CAD build for the part. Positions are in the model's coordinates, mm. A direction names the side the tool comes from. Coordinates: 2 decimals unless noted, no trailing zeros. Loops run counter-clockwise (first coordinate to the right, second up) from the corner with the lowest first, then second, coordinate; pieces in that order, holes last. Notation, with made-up numbers: (76, -33) -> (124, -33) arc R22 cw to (124, -5) -> close; hole circle Ø7 at (24.5, 20.25). An arc over 180 degrees is marked (long way). Return JSON: item names as keys, results as strings. Group by question number.
(1) Flat gauge pins, fed straight in: pin 1 Ø4 at (x, y) = (-8.5, -72.5) entering from +Z; pin 2 Ø12 at (x, y) = (-67.5, 66) entering from +Z; pin 3 Ø1 at (y, z) = (4.5, 59.5) entering from -X; pin 4 Ø4 at (x, y) = (-84.36, -38.25) entering from -Z. Where does each tip first touch, or does it go through?
(2) Saw through at B-B on x = 77. Write the cut outline in (y, z).
(3) Saw through at D-D on z = 54.25. Give the number of separate pieces and of enclosed holes in the cut face, then the cut area to 3 significant figures.
(4) Tool access for faces 1 (the face through (-72.5, 0, 57)), 2 (the face through (-77, 48, 57)): list every direction of +Z, -Z, +X, -X, +Y, -Y with a clear straight run to the whole face (end or side of a thin tool).
(5) Saw through at A-A on y = -13.5. Write the cut outline in (x, z), then the cut area to 3 significant figures.
(6) Mould opens along Y. For faces 3 (the face through (39.16, -61.41, 56.94)), 4 (the face through (-1.588, -84.596, 54.972)) say: pulls with the +Y half, pulls with the -Y half, needs draft (parallel to the pull), parting line crosses it, or undercut.
(7) Saw through at C-C on x = 22. Write the cut outline in (y, z).
(8) Probe L1, parallel to Y at x = 77.5, z = 60.5; L2, parallel to Y at x = -67.5, z = 55; L3, parallel to Y at x = -35, z = 56. List the from-to ranges inside material, lowest first.
```python
from build123d import *

# Parameters (mm, degrees)
F0_W      = 190
F0_H      = 175
F1_DEPTH  = 8
F2_R      = 4.5
F2_R_2    = 1.6
F3_DEPTH  = 8
F5_DEPTH  = 8.001
F6_R      = 12.2
F6_R_2    = 4.5
F7_DEPTH  = 4
F8_R      = 1.7
F8_W      = 145
F8_H      = 33.2
F8_R_2    = 1.8
F9_DEPTH  = 8.001
F10_ANGLE = 180


with BuildPart() as f1:
    # F0 (on Top) → F1 (new body)
    with BuildSketch(Plane.XY):
        Rectangle(F0_W, F0_H)
    extrude(amount=F1_DEPTH)

    # F2 (on face) → F3 (cut)
    with BuildSketch(Plane.XY.offset(8)):
        with Locations((0, 72.5)):
            Circle(F2_R)
        with Locations((-77, 42.5)):
            Circle(F2_R)
        with Locations((8.5, 72.5)):
            Circle(F2_R_2)
        with Locations((-8.5, 72.5)):
            Circle(F2_R_2)
        with Locations((-84.361216, 38.25)):
            Circle(F2_R_2)
        with Locations((-69.638784, 46.75)):
            Circle(F2_R_2)
        with Locations((77, 42.5)):
            Circle(F2_R)
        with Locations((84.361216, 38.25)):
            Circle(F2_R_2)
        with Locations((69.638784, 46.75)):
            Circle(F2_R_2)
        with Locations((-84.361216, -38.25)):
            Circle(F2_R_2)
        with Locations((-77, -42.5)):
            Circle(F2_R)
        with Locations((-69.638784, -46.75)):
            Circle(F2_R_2)
        with Locations((-8.5, -72.5)):
            Circle(F2_R_2)
        with Locations((0, -72.5)):
            Circle(F2_R)
        with Locations((8.5, -72.5)):
            Circle(F2_R_2)
        with Locations((69.638784, -46.75)):
            Circle(F2_R_2)
        with Locations((77, -42.5)):
            Circle(F2_R)
        with Locations((84.361216, -38.25)):
            Circle(F2_R_2)
    extrude(amount=-F3_DEPTH, mode=Mode.SUBTRACT)

    # F4 (on face) → F5 (cut, through all)
    with BuildSketch(Plane.XY.offset(8)):
        with BuildLine():
            Line((-64.009619, 50), (-15, 72.5))
            ThreePointArc((-15, 72.5), (-10.606602, 83.106602), (0, 87.5))
            Line((0, 87.5), (-95, 87.5))
            Line((-95, 87.5), (-95, -87.5))
            Line((-95, -87.5), (0, -87.5))
            ThreePointArc((0, -87.5), (-10.606602, -83.106602), (-15, -72.5))
            Line((-15, -72.5), (-64.009619, -50))
            ThreePointArc((-64.009619, -50), (-84.5, -55.490381), (-89.990381, -35))
            Line((-89.990381, -35), (-89.990381, 35))
            ThreePointArc((-89.990381, 35), (-84.5, 55.490381), (-64.009619, 50))
        make_face()
        with BuildLine():
            Line((95, 87.5), (0, 87.5))
            ThreePointArc((0, 87.5), (10.606602, 83.106602), (15, 72.5))
            Line((15, 72.5), (64.009619, 50))
            ThreePointArc((64.009619, 50), (84.5, 55.490381), (89.990381, 35))
            Line((89.990381, 35), (89.990381, -35))
            ThreePointArc((89.990381, -35), (84.5, -55.490381), (64.009619, -50))
            Line((64.009619, -50), (15, -72.5))
            ThreePointArc((15, -72.5), (10.606602, -83.106602), (0, -87.5))
            Line((0, -87.5), (95, -87.5))
            Line((95, -87.5), (95, 87.5))
        make_face()
    extrude(amount=-F5_DEPTH, mode=Mode.SUBTRACT)

    # F6 (on face) → F7 (cut)
    with BuildSketch(Plane.XY.offset(8)):
        with Locations((0, 72.5)):
            Circle(F6_R)
        with Locations((0, 72.5)):
            Circle(F6_R_2, mode=Mode.SUBTRACT)
        with Locations((-77, 42.5)):
            Circle(F6_R)
        with Locations((-77, 42.5)):
            Circle(F6_R_2, mode=Mode.SUBTRACT)
        with Locations((77, 42.5)):
            Circle(F6_R)
        with Locations((-77, -42.5)):
            Circle(F6_R)
        with Locations((0, -72.5)):
            Circle(F6_R)
        with Locations((77, -42.5)):
            Circle(F6_R)
    extrude(amount=-F7_DEPTH, mode=Mode.SUBTRACT)

    # F8 (on face) → F9 (cut, through all)
    with BuildSketch(Plane.XY.offset(8)):
        with Locations((0, 45)):
            Circle(F8_R)
        with Locations((0, 26.6)):
            Circle(F8_R)
        with Locations((-67.5, 26.6)):
            Circle(F8_R)
        with Locations((-35, 26.6)):
            Circle(F8_R)
        with Locations((35, 26.6)):
            Circle(F8_R)
        with Locations((67.5, 26.6)):
            Circle(F8_R)
        with Locations((67.5, -26.6)):
            Circle(F8_R)
        with Locations((35, -26.6)):
            Circle(F8_R)
        with Locations((0, -26.6)):
            Circle(F8_R)
        with Locations((0, -45)):
            Circle(F8_R)
        with Locations((-35, -26.6)):
            Circle(F8_R)
        with Locations((-67.5, -26.6)):
            Circle(F8_R)
        Rectangle(F8_W, F8_H)
        with Locations((-79.990381, 0)):
            Circle(F8_R_2)
    extrude(amount=-F9_DEPTH, mode=Mode.SUBTRACT)


with BuildPart() as f1_1:
    # F10: moved
    add(f1.part.rotate(Axis((0, 0, 0), (1, 0, 0)), F10_ANGLE))


with BuildPart() as f1_2:
    # F11: moved
    add(f1_1.part.moved(Location((0, 0, 56.2))))


with BuildPart() as f1_3:
    # F12: moved
    add(f1_2.part.moved(Location((0, 0, 4.8))))


solid = f1_3.part
```
Geometry results:
{
 "1": {"pin 1": "z = 61", "pin 2": "through", "pin 3": "x = -89.99", "pin 4": "z = 57"},
 "2": {"outline": "(-57.5, 53) -> (-54.7, 53) -> (-54.7, 57) -> (-47, 57) -> (-47, 61) -> (-57.5, 61) -> close; (-38, 57) -> (-30.3, 57) -> (-30.3, 53) -> (30.3, 53) -> (30.3, 57) -> (38, 57) -> (38, 61) -> (-38, 61) -> close; (47, 57) -> (54.7, 57) -> (54.7, 53) -> (57.5, 53) -> (57.5, 61) -> (47, 61) -> close"},
 "3": {"separate pieces": "1", "enclosed holes": "20", "area": "15,200 mm²"},
 "4": {"face 1": "+Z, -Z", "face 2": "-Z"},
 "5": {"outline": "(-89.99, 53) -> (-72.5, 53) -> (-72.5, 61) -> (-89.99, 61) -> close; (72.5, 53) -> (89.99, 53) -> (89.99, 61) -> (72.5, 61) -> close", "area": "280 mm²"},
 "6": {"face 3": "pulls with the -Y half", "face 4": "undercut"},
 "7": {"outline": "(-69.29, 53) -> (-16.6, 53) -> (-16.6, 61) -> (-69.29, 61) -> close; (16.6, 53) -> (69.29, 53) -> (69.29, 61) -> (16.6, 61) -> close"},
 "8": {"L1": "-57.49 to -46.97, -38.03 to 38.03, 46.97 to 57.49", "L2": "-54.11 to -50.15, -34.85 to -28.3, -24.9 to -16.6, 16.6 to 24.9, 28.3 to 34.85, 50.15 to 54.11", "L3": "-63.32 to -28.3, -24.9 to -16.6, 16.6 to 24.9, 28.3 to 63.32"}
}
